```python
from build123d import *

# Parameters (mm, degrees)
F1_DEPTH = 3
F2_R     = 3
F3_DEPTH = 24


# Not quite as in the source:
# - a feature names something its author has since deleted; it is built from what else it names


with BuildPart() as f1:
    # F0 (on Right) → F1 (new body)
    with BuildSketch(Plane.YZ):
        Polygon((5.7734155665, -0.0317179771), (2.9141763572, 4.9840655586), (-2.8592392093, 5.0157835357), (-5.7734155665, 0.0317179771), (-2.9141763572, -4.9840655586), (2.8592392093, -5.0157835357), align=None)
    extrude(amount=F1_DEPTH)

    # F2 (on face) → F3 (join)
    with BuildSketch(Plane(origin=(0, 0, 0), x_dir=(0, -1, 0), z_dir=(-1, 0, 0))):
        Circle(F2_R)
    extrude(amount=F3_DEPTH)


solid = f1.part
```
Input: part model. Units: mm. Frame: model coordinates. A direction names the side the tool comes from. Coordinates: 2 decimals unless noted, no trailing zeros. Order: outer loops, then holes, each group sorted by start corner. A loop starts at its lowest first (then second) coordinate and runs counter-clockwise, first axis right, second up. Notation, with made-up numbers: (-40, 51) - (9, 51) arc R19 cw to (9, 56) - close; hole circle Ø2 at (-28, 1.25). An arc over 180 degrees is marked (long way). Put each result on its own line as item: value.
1. Line query: line 1 along X through (y, z) = (-3, 4); line 2 along Y through (x, z) = (-4.25, 2.75); line 3 along Z through (x, y) = (-7.5, 1.75). Output: solid intervals per line, ascending.
Report:
line 1: x = 0 to 3
line 2: y = -1.2 to 1.2
line 3: z = -2.44 to 2.44
2. Contact query for flat-ended pins moving along their axis: pin 1 Ø2 at (x, y) = (-8.5, -1.5) entering from -Z; pin 2 Ø3 at (x, z) = (-2, -4) entering from +Y; pin 3 Ø6 at (x, z) = (-16, 3.5) entering from -Y. Output: stop coordinate, or through.
Report:
pin 1: stops at z = -2.96
pin 2: stops at y = 1.66
pin 3: stops at y = -2.96
3. Cut plane C-C on x = -14.5. Return the cut outline in (y, z).
Report:
outline: circle Ø6 at (0, 0)
4. Cut plane D-D on y = 3.5. Return the cut outline in (x, z).
Report:
outline: (0, -3.92) - (3, -3.92) - (3, 3.96) - (0, 3.96) - close
5. Reachability of faces 1 (the face through (-12, 3, 0)), 2 (the face through (-24, 0, 0)) from +Z, -Z, +X, -X, +Y, -Y: full face, straight path, thin tool, end or side. Return the list, or none.
Report:
face 1: -X
face 2: +Z, -Z, -X, +Y, -Y
6. Cut plane B-B on z = -0.5. Return the cut outline in (x, y).
Report:
outline: (-24, -2.96) - (0, -2.96) - (0, -5.47) - (3, -5.47) - (3, 5.5) - (0, 5.5) - (0, 2.96) - (-24, 2.96) - close
7. Cut plane A-A on y = 0. Return the cut outline in (x, z).
Report:
outline: (-24, -3) - (0, -3) - (0, -5) - (3, -5) - (3, 5) - (0, 5) - (0, 3) - (-24, 3) - close
